Part model, mm, in its own coordinate system. A direction names the side the tool comes from. Coordinates: 2 decimals unless noted, no trailing zeros. Order: outer loops, then holes, each group sorted by start corner. A loop starts at its lowest first (then second) coordinate and runs counter-clockwise, first axis right, second up.
from build123d import *

# Parameters (mm, degrees)
SKETCH3_R               = 3.917718569
SKETCH3_R_2             = 3.6195
CUT_EXTRUDE1_DEPTH      = 16.51
CUT_EXTRUDE2_DEPTH      = 86.489963921
CUT_EXTRUDE2_DEPTH_BACK = 86.489963921
CUT_EXTRUDE3_DEPTH      = 86.489963921
CUT_EXTRUDE3_DEPTH_BACK = 86.489963921
FILLET1_R               = 0.635


with BuildPart() as part:
    # Sweep1: sweep along a path in Sketch1
    with BuildLine(Plane(origin=(0, 0, 0), x_dir=(1, 0, 0), z_dir=(0, 1, 0))) as sweep1_path:
        Line((0, 0), (-60.1218, 0))
        ThreePointArc((-60.1218, 0), (-77.7748, 17.653), (-60.1218, 35.306))
        Line((-60.1218, 35.306), (-16.3068, 35.306))
    # Sketch2 → Sweep1 (sweep)
    with BuildSketch(Plane(origin=(0, 0, 0), x_dir=(0, 0, -1), z_dir=(1, 0, 0))):
        Polygon((7.239, 1.499245989), (5.118745989, 3.6195), (2.120254011, 3.6195), (0, 1.499245989), (0, -1.499245989), (2.120254011, -3.6195), (5.118745989, -3.6195), (7.239, -1.499245989), align=None)
    sweep(path=sweep1_path.line)

    # Sketch3 → Cut-Extrude1 (cut)
    with BuildSketch(Plane(origin=(0, 0, 0), x_dir=(0, 0, -1), z_dir=(1, 0, 0))):
        with Locations((3.6195, 0)):
            Circle(SKETCH3_R)
        with Locations((3.6195, 0)):
            Circle(SKETCH3_R_2, mode=Mode.SUBTRACT)
    extrude(amount=-CUT_EXTRUDE1_DEPTH, mode=Mode.SUBTRACT)

    # Sketch5 → Cut-Revolve1 (revolve, cut)
    with BuildSketch(Plane(origin=(0, 0, 0), x_dir=(1, 0, 0), z_dir=(0, 1, 0))):
        with BuildLine():
            Line((-8.255, 7.239), (-3.175, 7.239))
            ThreePointArc((-3.175, 7.239), (-5.715, 6.096), (-8.255, 7.239))
        make_face()
    revolve(axis=Axis((0, 0, -3.6195), (-1, 0, 0)), mode=Mode.SUBTRACT)

    # Sketch6 → Cut-Extrude2 (cut, two sides: drawn at the far end of the back side and taken through both)
    with BuildSketch(Plane(origin=(0, 0, 0), x_dir=(1, 0, 0), z_dir=(0, 1, 0)).offset(-CUT_EXTRUDE2_DEPTH_BACK)):
        with BuildLine():
            Line((-18.8468, 28.067), (-26.4668, 28.067))
            ThreePointArc((-26.4668, 28.067), (-22.6568, 30.607), (-18.8468, 28.067))
        make_face()
        with BuildLine():
            Line((-18.8468, 7.239), (-26.4668, 7.239))
            ThreePointArc((-26.4668, 7.239), (-22.6568, 4.699), (-18.8468, 7.239))
        make_face()
    extrude(amount=CUT_EXTRUDE2_DEPTH + CUT_EXTRUDE2_DEPTH_BACK, mode=Mode.SUBTRACT)

    # Sketch7 → Cut-Extrude3 (cut, two sides: drawn at the far end of the back side and taken through both)
    with BuildSketch(Plane(origin=(0, 0, 0), x_dir=(1, 0, 0), z_dir=(0, 1, 0)).offset(-CUT_EXTRUDE3_DEPTH_BACK)):
        with BuildLine():
            Line((-5.715, 6.096), (-19.561541368, 6.096))
            ThreePointArc((-19.561541368, 6.096), (-19.157191244, 6.638122792), (-18.8468, 7.239))
            Line((-18.8468, 7.239), (-8.255, 7.239))
            ThreePointArc((-8.255, 7.239), (-7.107663725, 6.394913945), (-5.715, 6.096))
        make_face()
    extrude(amount=CUT_EXTRUDE3_DEPTH + CUT_EXTRUDE3_DEPTH_BACK, mode=Mode.SUBTRACT)

    # Fillet1
    fillet1_edges = [part.edges().sort_by_distance(p)[0] for p in [
        (-16.3068, 0, -28.067),
        (-16.3068, 2.559372995, -29.127127005),
        (-16.3068, 3.6195, -31.6865),
        (-16.3068, 2.559372995, -34.245872995),
        (-16.3068, 0, -35.306),
        (-16.3068, -2.559372995, -34.245872995),
        (-16.3068, -3.6195, -31.6865),
        (-16.3068, -2.559372995, -29.127127005),
        (0, 0, 0),
    ]]
    fillet(fillet1_edges, radius=FILLET1_R)


solid = part.part
Q1. Mould opens along Z. For faces 4 (the face through (-75.99, -3.28, -17.3)), 5 (the face through (-43, 0, -28.067)), 6 (the face through (-38.23, -2.545, -34.261)) say: pulls with the +Z half, pulls with the -Z half, needs draft (parallel to the pull), parting line crosses it, or undercut.
Results list:
face 4: parting line crosses it
face 5: undercut
face 6: pulls with the -Z half
Q2. Wall check: line 1 along Z through (x, y) = (-53.5, -0.75); line 2 along Z through (x, y) = (-23, -0.75); line 3 along X through (y, z) = (0, -28.5). Give the ranges that are in metal, low to high.
Results list:
line 1: z = -35.31 to -28.07, -7.24 to 0
line 2: z = -35.31 to -30.59, -4.71 to 0
line 3: x = -74.05 to -26.26, -19.06 to -16.34
Q3. Pin check, flat tips, straight feed: pin 1 Ø0.8 at (y, z) = (-3, -5.5) entering from +X; pin 2 Ø4 at (x, y) = (-11, 0.5) entering from -Z; pin 3 Ø1.8 at (y, z) = (-0.5, -33) entering from +X. Stop position of each tip, or through.
Results list:
pin 1: stops at x = -0.02
pin 2: stops at z = -6.1
pin 3: stops at x = -16.31
Q4. Which spindle directions (+Z, -Z, +X, -X, +Y, -Y) get a long thin tool onto all of the face, cutting with end or side? Do faces 1 (the face through (-16.488, -2.41, -29.247)), 2 (the face through (-16.5, 2.45, -29.27)), 3 (the face through (-1.89, 1.09, -7.07)). Say none if no direction does.
Results list:
face 1: +X, -Y
face 2: +X, +Y
face 3: +X
Q5. Cut at A-A on x = -39. Write the cut outline in (y, z), and give its area (3 significant figures).
Results list:
outline: (-3.62, -33.19) - (-1.5, -35.31) - (1.5, -35.31) - (3.62, -33.19) - (3.62, -30.19) - (1.5, -28.07) - (-1.5, -28.07) - (-3.62, -30.19) - close; (-3.62, -5.12) - (-1.5, -7.24) - (1.5, -7.24) - (3.62, -5.12) - (3.62, -2.12) - (1.5, 0) - (-1.5, 0) - (-3.62, -2.12) - close
area: 86.8 mm2
